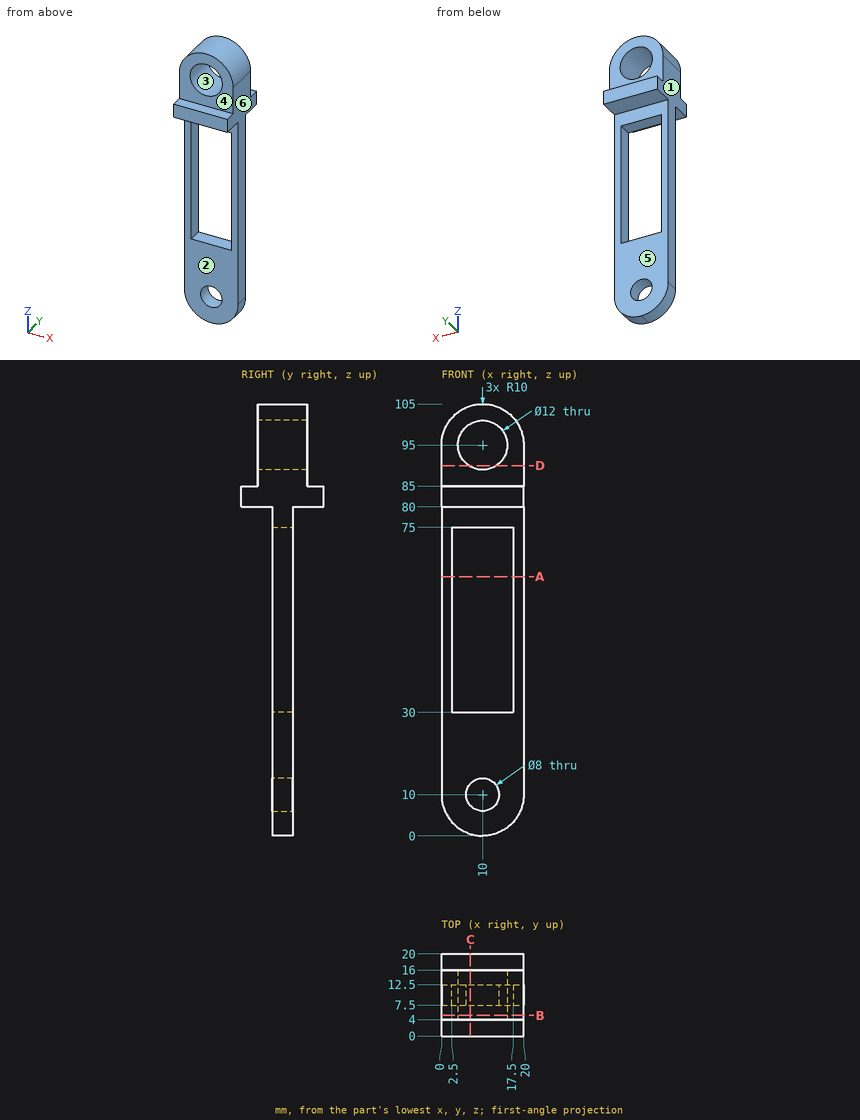
The figure shows three views and two pictorial views of one solid part (mm, origin at its lowest corner). Answer the questions. A direction names the side the tool comes from. Coordinates: 2 decimals unless noted, no trailing zeros. Loops run counter-clockwise (first coordinate to the right, second up) from the corner with the lowest first, then second, coordinate; pieces in that order, holes last. Notation, with made-up numbers: (-28, 51.25) - (-17, 51.25) arc R21 cw to (-17, 82.25) - close; hole circle Ø2 at (-37.5, 38). An arc over 180 degrees is marked (long way). Use a Markdown table: item, result. Add a question column.
1) The part is cut by section A-A, the plane z = 63. Give the vertices of the cut face in (x, y).
2) The part is cut by section C-C, the plane x = 7. Give the vertices of the cut face in (y, z), and give its area (3 significant figures).
3) The part is cut by section D-D, the plane z = 90. Give the vertices of the cut face in (x, y), and give its area (3 significant figures).
4) The mould has two halves that part along X. Classify the marked faces 1, 2 and 3: released by +X, released by -X, zero draft, split by the parting line, or undercut.
5) Given pin 1 (4 mm diameter, centred on x = 8.5, y = 3.5, fed in from -Z); pin 2 (4 mm diameter, centred on x = 8.5, y = 9, fed in from +Z); pin 3 (8 mm diameter, centred on y = 2.5, z = 14.5, fed in from -X); pin 4 (12 mm diameter, centred on x = 14.5, z = 32, fed in from +Y), each flat-ended and moving along its own axis, determine where each tip first touches the part or whether it passes through.
6) Find the intervals of material crossed by line 1 (X direction, y = 10.35, z = 10); line 2 (X direction, y = 12, z = 95); line 3 (Z direction, x = 6.5, y = 2), in increasing order.
7) The part is cut by section B-B, the plane y = 5. Give the vertices of the cut face in (x, z).
8) For the marked faces 4, 5 and 6, determine the directions among +Z, -Z, +X, -X, +Y, -Y from which every point of the face is accessible in a straight line to the end or side of a thin tool.
Here are the results:
| question | item | result |
|---|---|---|
| 1 | outline | (0, 7.5) - (2.5, 7.5) - (2.5, 12.5) - (0, 12.5) - close; (17.5, 7.5) - (20, 7.5) - (20, 12.5) - (17.5, 12.5) - close |
| 2 | outline | (0, 80) - (7.5, 80) - (7.5, 75) - (12.5, 75) - (12.5, 80) - (20, 80) - (20, 85) - (16, 85) - (16, 89.8) - (4, 89.8) - (4, 85) - (0, 85) - close; (4, 100.2) - (16, 100.2) - (16, 104.54) - (4, 104.54) - close; (7.5, 0.46) - (12.5, 0.46) - (12.5, 7.35) - (7.5, 7.35) - close; (7.5, 12.65) - (12.5, 12.65) - (12.5, 30) - (7.5, 30) - close |
| 2 | area | 356 mm^2 |
| 3 | outline | (0, 4) - (6.68, 4) - (6.68, 16) - (0, 16) - close; (13.32, 4) - (20, 4) - (20, 16) - (13.32, 16) - close |
| 3 | area | 160 mm^2 |
| 4 | face 1 | released by -X |
| 4 | face 2 | zero draft |
| 4 | face 3 | undercut |
| 5 | pin 1 | stops at z = 80 |
| 5 | pin 2 | stops at z = 105 |
| 5 | pin 3 | passes through |
| 5 | pin 4 | stops at y = 12.5 |
| 6 | line 1 | x = 0 to 6, 14 to 20 |
| 6 | line 2 | x = 0 to 4, 16 to 20 |
| 6 | line 3 | z = 80 to 85 |
| 7 | outline | (0, 80) - (20, 80) - (20, 95) arc R10 ccw to (0, 95) - close; hole circle Ø12 at (10, 95) |
| 8 | face 4 | +Z, +X, -X, -Y |
| 8 | face 5 | -Z, +X, -X, +Y |
| 8 | face 6 | +Z, -Z, +X, +Y, -Y |
